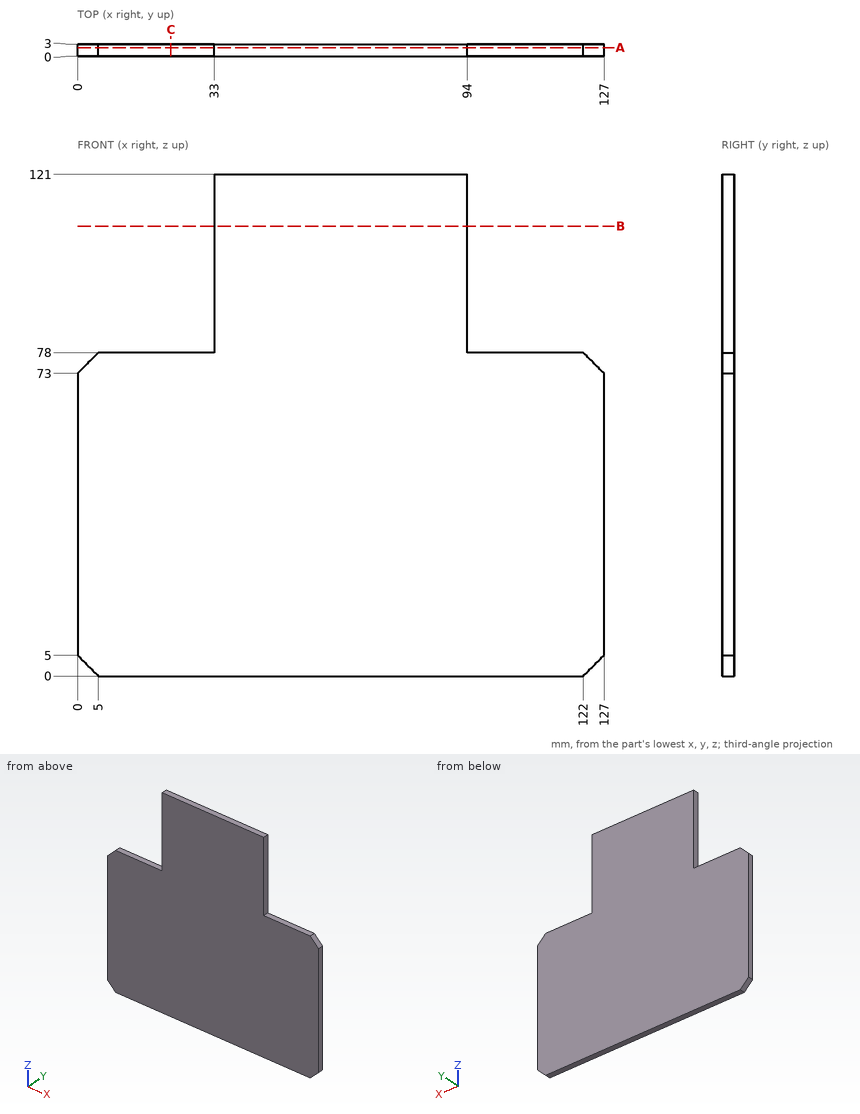
Part print with two shaded views. Sizes in mm from the minimum x, y, z corner. Round coordinates to 2 decimals unless told otherwise and drop trailing zeros. Loops run counter-clockwise (first coordinate to the right, second up) from the corner with the lowest first, then second, coordinate; pieces in that order, holes last. Notation, with made-up numbers: (74, 37.5) - (107, 37.5) arc R10 ccw to (107, 44.5) - close; hole circle Ø10 at (71.25, 87). An arc over 180 degrees is marked (long way). Answer as a JSON object with one key per item and string values.
Item 1: Pin check, flat tips, straight feed: pin 1 (0.9 mm diameter, centred on x = 12.5, y = 1.5, fed in from +Z); pin 2 (1.5 mm diameter, centred on y = 1.5, z = 92, fed in from -X). Stop position of each tip, or through.
Output:
{"pin 1": "z = 78", "pin 2": "x = 33"}
Item 2: Band-saw the part on A-A on y = 2.15. List the corners of the cut face in (x, z).
Output:
{"outline": "(0, 5) - (5, 0) - (122, 0) - (127, 5) - (127, 73) - (122, 78) - (94, 78) - (94, 121) - (33, 121) - (33, 78) - (5, 78) - (0, 73) - close"}
Item 3: Wall check: L1, parallel to X at y = 1.05, z = 88; L2, parallel to Z at x = 9.5, y = 0.4; L3, parallel to X at y = 2.9, z = 74.5. Give the ranges that are in metal, low to high.
Output:
{"L1": "33 to 94", "L2": "0 to 78", "L3": "1.5 to 125.5"}
Item 4: Band-saw the part on B-B on z = 108.5. List the corners of the cut face in (x, y), plus the area to 3 significant figures.
Output:
{"outline": "(33, 0) - (94, 0) - (94, 3) - (33, 3) - close", "area": "183 mm2"}
Item 5: Band-saw the part on C-C on x = 22.5. List the corners of the cut face in (y, z).
Output:
{"outline": "(0, 0) - (3, 0) - (3, 78) - (0, 78) - close"}
